Source: three-view drawing plus pictorial views. Frame: mm from the lowest corner of the part. Round coordinates to 2 decimals unless told otherwise and drop trailing zeros. Loops run counter-clockwise (first coordinate to the right, second up) from the corner with the lowest first, then second, coordinate; pieces in that order, holes last. Notation, with made-up numbers: M 52,-10 L 88,-10 A35 ccw 88,26 Z; hole C -26,38.25 d5. An arc over 180 degrees is marked long. Answer as a JSON object with one key per item and string values.
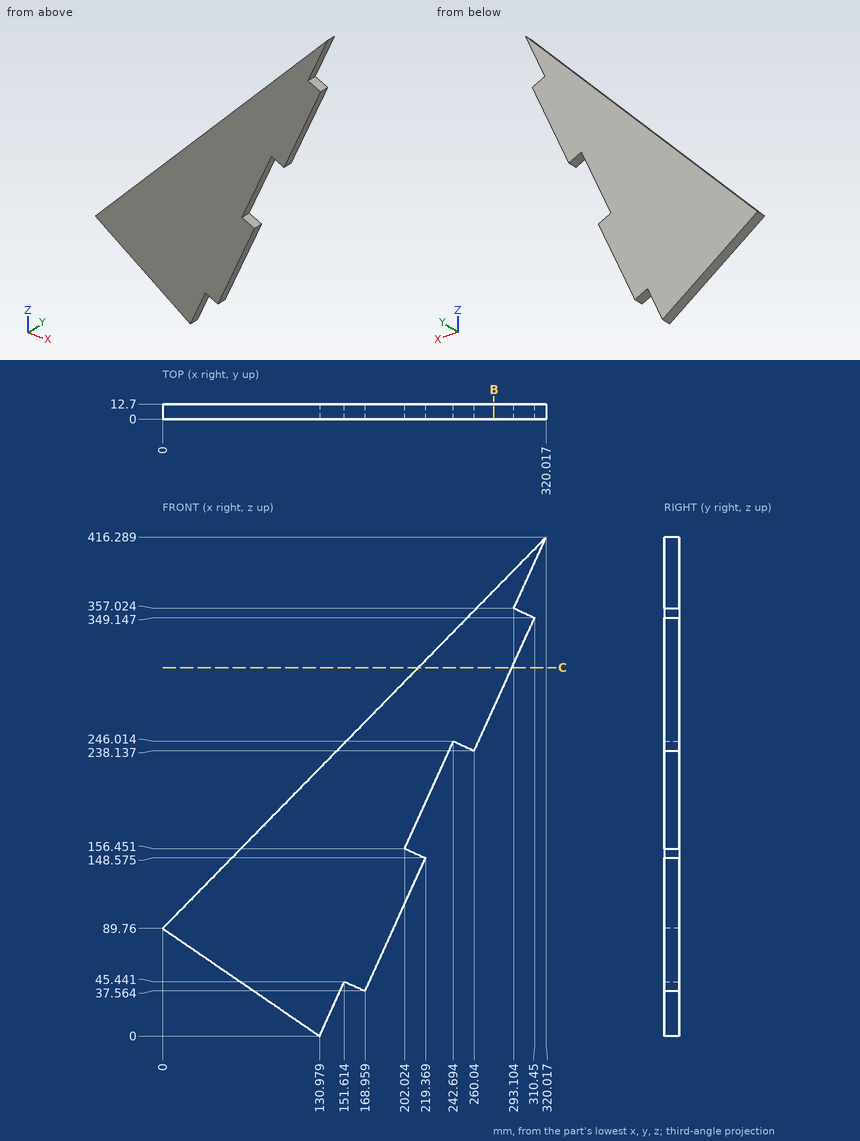
1) Cut plane C-C on z = 307.5. Return the cut outline in (x, y).
Geometry results:
{"outline": "M 213.4,0 L 291.54,0 L 291.54,12.7 L 213.4,12.7 Z"}
2) Line query: probe 1 along Z at (x, y) = (30.5, 6); probe 2 along Z at (x, y) = (160, 5.75) (1 decimal); probe 3 along X at (y, z) = (5, 353) (1 decimal). Output: solid intervals per line, ascending.
Geometry results:
{"probe 1": "68.86 to 120.88", "probe 2": "41.6 to 253", "probe 3": "258 to 302"}
3) First-contact query: pin 1 (3 mm diameter, centred on y = 7.5, z = 123.5, fed in from +X) (1 decimal); pin 2 (2 mm diameter, centred on y = 3.5, z = 349, fed in from +X); pin 3 (5 mm diameter, centred on y = 8.5, z = 324, fed in from -X). Flat tips, straight axial feed; report the tip coordinate or a pass-through.
Geometry results:
{"pin 1": "x = 208.7", "pin 2": "x = 310.45", "pin 3": "x = 227.12"}
4) Cut plane B-B on x = 276.5. Return the cut outline in (y, z) (1 decimal), and give its area (3 significant figures).
Geometry results:
{"outline": "M 0,274.4 L 12.7,274.4 L 12.7,371.9 L 0,371.9 Z", "area": "1,240 mm2"}
